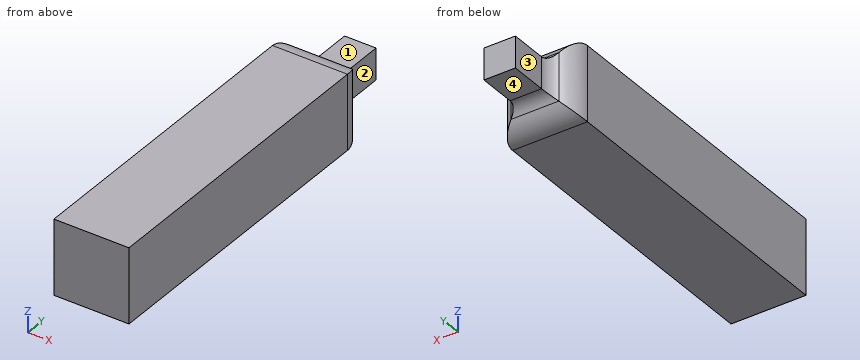
```python
from build123d import *

# Parameters (mm, degrees)
SKETCH1_W           = 15.5
SKETCH1_H           = 15.5
BOSS_EXTRUDE1_DEPTH = 70
SKETCH2_W           = 6.5
SKETCH2_H           = 6.5
BOSS_EXTRUDE2_DEPTH = 10
FILLET1_R           = 5
FILLET2_R           = 3


with BuildPart() as part:
    # Sketch1 → Boss-Extrude1 (new body)
    with BuildSketch(Plane(origin=(0, 0, 0), x_dir=(1, 0, 0), z_dir=(0, 1, 0))):
        Rectangle(SKETCH1_W, SKETCH1_H)
    extrude(amount=BOSS_EXTRUDE1_DEPTH)

    # Sketch2 → Boss-Extrude2 (add)
    with BuildSketch(Plane(origin=(0, 70, 0), x_dir=(1, 0, 0), z_dir=(0, 1, 0))):
        Rectangle(SKETCH2_W, SKETCH2_H)
    extrude(amount=BOSS_EXTRUDE2_DEPTH)

    # Fillet1
    # the kernel refuses this fillet: 5 mm, written as the material it takes off along each edge
    with BuildSketch(Plane(origin=(-7.75, 70, 20.187342964), x_dir=(0, -1, 0), z_dir=(0, 0, -1)), Plane(origin=(7.75, 70, -20.187342964), x_dir=(0, -1, 0), z_dir=(0, 0, 1)), Plane(origin=(-20.187342964, 70, -7.75), x_dir=(0, -1, 0), z_dir=(1, 0, 0))) as fillet1_piece_1:
        with BuildLine():
            CenterArc((4.974937186, -5), FILLET1_R, 90, 84.260829523)
            Line((0, -4.5), (-0.099498744, -4.49))
            ThreePointArc((-0.099498744, -4.49), (-0.1, -2.25), (-0.1, 0))
            Line((-0.1, 0), (0, 0.1))
            Line((0, 0.1), (4.974937186, 0.1))
            Line((4.974937186, 0.1), (4.974937186, 0))
        make_face()
    extrude(amount=40.374685928, mode=Mode.SUBTRACT)
    with BuildSketch(Plane(origin=(20.187342964, 70, 7.75), x_dir=(0, 0, -1), z_dir=(-1, 0, 0))) as fillet1_piece_2:
        with BuildLine():
            CenterArc((5, 4.974937186), FILLET1_R, 180, 84.260829523)
            Line((0, 4.974937186), (-0.1, 4.974937186))
            Line((-0.1, 4.974937186), (-0.1, 0))
            Line((-0.1, 0), (0, -0.1))
            ThreePointArc((0, -0.1), (2.25, -0.1), (4.49, -0.099498744))
            Line((4.49, -0.099498744), (4.5, 0))
        make_face()
    extrude(amount=40.374685928, mode=Mode.SUBTRACT)

    # Fillet2
    fillet2_edges = [part.edges().sort_by_distance(p)[0] for p in [
        (-3.25, 70, 0),
        (0, 70, -3.25),
        (0, 70, 3.25),
        (3.25, 70, 0),
    ]]
    fillet(fillet2_edges, radius=FILLET2_R)


solid = part.part
```
Design review of the part built by this model. Coordinates are the model's own, in mm. Face numbers are marked on the shaded views. A direction names the side the tool comes from. Coordinates: 2 decimals unless noted, no trailing zeros. Write each loop counter-clockwise with the first axis right and the second up, starting at its lowest first coordinate (ties: lowest second). Pieces come first, ordered by that corner, then holes.
1) Machinability: for the marked faces 1, 2, 3 and 4, which of the approach directions +Z, -Z, +X, -X, +Y, -Y give a long, thin tool a straight path to every point of the face, cutting with its end or side? Answer none if there is none.
2) Insertion check: pin 1 (5 mm diameter, centred on y = 76.5, z = -0.5, fed in from -X); pin 2 (3 mm diameter, centred on y = 75, z = -1.5, fed in from +X); pin 3 (7 mm diameter, centred on x = -1, y = 76.5, fed in from +Z). Each pin has a flat end and moves straight along its axis. Give the tip position at first contact, or say it passes through.
3) Add section A-A (z = 2.5). Write out the cut boundary in (x, y), plus the area to 3 significant figures.
4) Add section B-B (x = 0.75). Write out the cut boundary in (y, z), plus the area to 3 significant figures.
5) Add section D-D (z = -6). Write out the cut boundary in (x, y), plus the area to 3 significant figures.
6) To check wall thickness, follow L1, parallel to Z at x = 2.5, y = 73; L2, parallel to Y at x = -0.75, z = 3.75. State the ranges of each line that lie inside material, in increasing order.
7) Add section C-C (x = 4). Write out the cut boundary in (y, z), plus the area to 3 significant figures.
Check result:
1. face 1: +Z, +X, -X, +Y
1. face 2: +Z, -Z, +X, +Y
1. face 3: +Z, -Z, -X, +Y
1. face 4: -Z, +X, -X, +Y
2. pin 1: stops at x = -3.25
2. pin 2: stops at x = 3.25
2. pin 3: stops at z = 3.25
3. outline: (-7.75, 0) - (7.75, 0) - (7.75, 65.03) arc R5 ccw to (4.94, 69.52) arc R3 cw to (3.25, 72.22) - (3.25, 80) - (-3.25, 80) - (-3.25, 72.22) arc R3 cw to (-4.94, 69.52) arc R5 ccw to (-7.75, 65.03) - close
3. area: 1,140 mm2
4. outline: (0, -7.75) - (65.03, -7.75) arc R5 ccw to (69.52, -4.94) arc R3 cw to (72.22, -3.25) - (80, -3.25) - (80, 3.25) - (72.22, 3.25) arc R3 cw to (69.52, 4.94) arc R5 ccw to (65.03, 7.75) - (0, 7.75) - close
4. area: 1,140 mm2
5. outline: (-7.75, 0) - (7.75, 0) - (7.75, 65.03) arc R5 ccw to (6, 68.82) - (-6, 68.82) arc R5 ccw to (-7.75, 65.03) - close
5. area: 1,060 mm2
6. L1: z = -3.25 to 3.25
6. L2: y = 0 to 70.56
7. outline: (0, -7.75) - (65.03, -7.75) arc R5 ccw to (69.52, -4.94) arc R3 cw to (70.23, -4) - (70.23, 4) arc R3 cw to (69.52, 4.94) arc R5 ccw to (65.03, 7.75) - (0, 7.75) - close
7. area: 1,080 mm2
